Job drawing, mm, ordinate dimensions from the low corner. One solid piece. A direction names the side the tool comes from. Coordinates: 2 decimals unless noted, no trailing zeros. Loops run counter-clockwise (first coordinate to the right, second up) from the corner with the lowest first, then second, coordinate; pieces in that order, holes last. Notation, with made-up numbers: (-6.5, 11) - (15.5, 11) arc R10 ccw to (15.5, 30) - close; hole circle Ø8 at (10.25, 15.25). An arc over 180 degrees is marked (long way). Use a Markdown table: item, result. Add a question column.
1. Drop flat-ended pins along their axis: pin 1 (6 mm diameter, centred on y = 7, z = 10.5, fed in from -X); pin 2 (22 mm diameter, centred on y = 29, z = 18.5, fed in from +X); pin 3 (1.5 mm diameter, centred on y = 23, z = 14, fed in from -X). Give the stop position or say it passes through.
2. 3-axis set-ups, long thin cutter, end or side, ignore diameter. For the marked faces 1 and 2: which of +Z, -Z, +X, -X, +Y, -Y reach the whole face in a straight line?
3. Band-saw the part on C-C, the plane z = 35.5. Give the cut face in (x, y), plus the area to 3 significant figures.
4. Band-saw the part on D-D, the plane y = 32.5. Give the cut face in (x, z).
5. Wall check: probe 1 along Y at (x, z) = (20, 5); probe 2 along Y at (x, z) = (60, 46); probe 3 along X at (y, z) = (17, 4.5). Give the ranges that are in metal, low to high. Write a range as [from, to].
6. Band-saw the part on B-B, the plane x = 60.5. Give the cut face in (y, z), plus the area to 3 significant figures.
7. Band-saw the part on A-A, the plane y = 24. Give the cut face in (x, z), plus the area to 3 significant figures.
8. Pull direction X, two halves, no side cores. Call the marked faces 3, 4, 5 and 6: pulls with the +X half, pulls with the -X half, needs draft (parallel to the pull), parting line crosses it, or undercut.
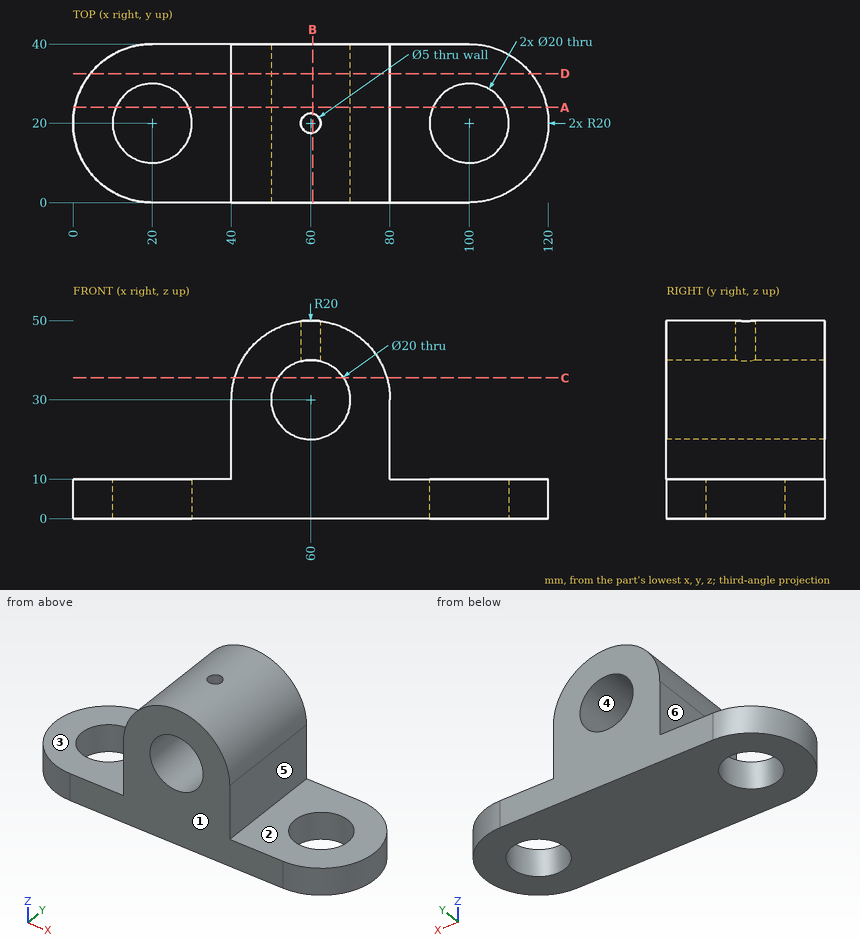
Geometry check:
| question | item | result |
|---|---|---|
| 1 | pin 1 | stops at x = 2.7 |
| 1 | pin 2 | stops at x = 119.9 |
| 1 | pin 3 | stops at x = 40 |
| 2 | face 1 | +Z, -Z, +X, -X, -Y |
| 2 | face 2 | +Z, +X, +Y, -Y |
| 3 | outline | (40.77, 0) - (51.65, 0) - (51.65, 40) - (40.77, 40) - close; (68.35, 0) - (79.23, 0) - (79.23, 40) - (68.35, 40) - close |
| 3 | area | 870 mm^2 |
| 4 | outline | (4.39, 0) - (115.61, 0) - (115.61, 10) - (80, 10) - (80, 30) arc R20 ccw to (40, 30) - (40, 10) - (4.39, 10) - close; hole circle Ø20 at (60, 30) |
| 5 | probe 1 | y = [0, 10], [30, 40] |
| 5 | probe 2 | y = [0, 17.5], [22.5, 40] |
| 5 | probe 3 | x = [0.23, 10.46], [29.54, 90.46], [109.54, 119.77] |
| 6 | outline | (0, 0) - (40, 0) - (40, 20.01) - (0, 20.01) - close; (0, 39.99) - (17.55, 39.99) - (17.55, 49.99) - (0, 49.99) - close; (22.45, 39.99) - (40, 39.99) - (40, 49.99) - (22.45, 49.99) - close |
| 6 | area | 1,150 mm^2 |
| 7 | outline | (0.4, 0) - (10.83, 0) - (10.83, 10) - (0.4, 10) - close; (29.17, 0) - (90.83, 0) - (90.83, 10) - (80, 10) - (80, 30) arc R20 ccw to (40, 30) - (40, 10) - (29.17, 10) - close; (109.17, 0) - (119.6, 0) - (119.6, 10) - (109.17, 10) - close; hole circle Ø20 at (60, 30) |
| 7 | area | 1,940 mm^2 |
| 8 | face 3 | needs draft |
| 8 | face 4 | undercut |
| 8 | face 5 | pulls with the +X half |
| 8 | face 6 | pulls with the -X half |
